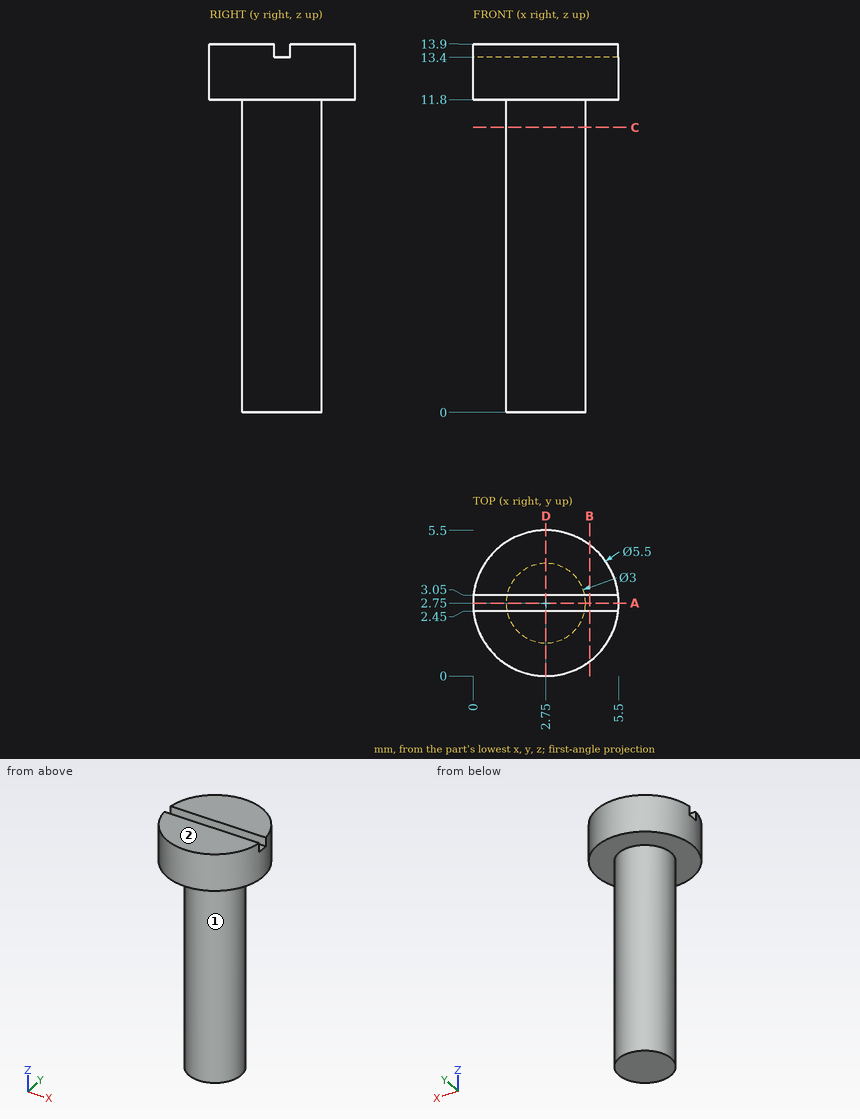
Study the drawing (mm; zero at the part's minimum x, y, z) and answer. A direction names the side the tool comes from. Give positions to 0.01 mm unless a question says otherwise; leave off trailing zeros. Write each loop counter-clockwise with the first axis right and the second up, starting at its lowest first coordinate (ties: lowest second). Pieces come first, ordered by that corner, then holes. Notation, with made-up numbers: (47, -20.5) -> (97, -20.5) arc R17 cw to (97, -9.5) -> close; hole circle Ø9 at (86, 56.5). An arc over 180 degrees is marked (long way). Answer as a JSON object with one key per item and string values. Group by question number.
1) Each of these flat-tipped pins is pushed along its axis until it touches: P1, Ø3, axis at x = 1, z = 10.5, coming from the +Y side; P2, Ø2, axis at x = 4.5, z = 10.5, coming from the -Y side; P3, Ø2, axis at y = 2, z = 3.5, coming from the -X side. Where does it stop, or does it pass through?
2) Consider L1, parallel to Z at x = 0.7, y = 1.6; L2, parallel to Z at x = 4.15, y = 2.6; L3, parallel to Y at x = 1.65, z = 7.75. Determine where each line is inside the solid, lowest interval first. Write a range as from..to.
3) Find section D-D (x = 2.75). Write down the section's boundary in (y, z).
4) Find section B-B (x = 4.4). Write down the section's boundary in (y, z).
5) Find section A-A (y = 2.75). Write down the section's boundary in (x, z).
6) A tool of negligible diameter and unlimited length cuts with its end or side. For the marked faces 1 and 2, from which of +Z, -Z, +X, -X, +Y, -Y can it reach the whole face along a straight path? Write none if from no direction.
7) Find section C-C (z = 10.75). Write down the section's boundary in (x, y), and give its area (3 significant figures).
Values follow:
{
 "1": {"P1": "stops at y = 5.31", "P2": "stops at y = 1.45", "P3": "stops at x = 1.25"},
 "2": {"L1": "z = 11.8..13.9", "L2": "z = 0..13.4", "L3": "y = 1.73..3.77"},
 "3": {"outline": "(0, 11.8) -> (1.25, 11.8) -> (1.25, 0) -> (4.25, 0) -> (4.25, 11.8) -> (5.5, 11.8) -> (5.5, 13.9) -> (3.05, 13.9) -> (3.05, 13.4) -> (2.45, 13.4) -> (2.45, 13.9) -> (0, 13.9) -> close"},
 "4": {"outline": "(0.55, 11.8) -> (4.95, 11.8) -> (4.95, 13.9) -> (3.05, 13.9) -> (3.05, 13.4) -> (2.45, 13.4) -> (2.45, 13.9) -> (0.55, 13.9) -> close"},
 "5": {"outline": "(0, 11.8) -> (1.25, 11.8) -> (1.25, 0) -> (4.25, 0) -> (4.25, 11.8) -> (5.5, 11.8) -> (5.5, 13.4) -> (0, 13.4) -> close"},
 "6": {"face 1": "-Z", "face 2": "+Z, +X, -X, +Y, -Y"},
 "7": {"outline": "circle Ø3 at (2.75, 2.75)", "area": "7.07 mm2"}
}
